Autodesk Inventor part; units mm, degrees
ref_plane "YZ Plane" through (0, 0, 0) normal (1, 0, 0) x (0, 1, 0)
ref_plane "XZ Plane" through (0, 0, 0) normal (0, 1, 0) x (-1, 0, 0)
ref_plane "XY Plane" through (0, 0, 0) normal (0, 0, 1) x (1, 0, 0)
sketch "Sketch1" plane through (0, 0, 0) normal (0, 1, 0) x (-1, 0, 0)
  line L0 (0, 0) -> (-27, 0) construction
  line L1 (-27, -8) -> (0, -8)
  arc A0 (0, -8) -> (0, 8) centre (0, 0) ccw
  arc A1 (-27, 8) -> (-27, -8) centre (-27, 0) ccw
  line L2 (14.5, 10) -> (-41.5, 10)
  line L3 (-41.5, 10) -> (-41.5, -10)
  line L4 (-41.5, -10) -> (14.5, -10)
  line L5 (14.5, -10) -> (14.5, 10)
  line L6 (14.5, 10) -> (-41.5, -10) construction
  line L7 (-41.5, 10) -> (14.5, -10) construction
  line L8 (14.5, 10) -> (-41.5, 10)
  line L9 (-41.5, 10) -> (-41.5, 15)
  line L10 (-41.5, 15) -> (14.5, 15)
  line L11 (14.5, 15) -> (14.5, 10)
  arc A2 (0, -8) -> (-5.3358, 5.9607) centre (0, 0) ccw
  arc A3 (-21.6642, 5.9607) -> (-27, -8) centre (-27, 0) ccw
  line L12 (9, -10) -> (-36, -10)
  line L13 (-36, -10) -> (-36, 10) construction
  line L14 (-36, 10) -> (9, 10)
  line L15 (9, 10) -> (9, -10) construction
  line L16 (9, -10) -> (-36, 10) construction
  line L17 (-36, -10) -> (9, 10) construction
  line L18 (9, 10) -> (-6, 10)
  line L19 (-6, 10) -> (-6, 5.9607)
  line L20 (-36, 10) -> (-21, 10)
  line L21 (-21, 10) -> (-21, 5.9607)
  line L22 (-5.3358, 5.9607) -> (-21.6642, 5.9607) construction
  line L23 (-21, 5.9607) -> (-21.6642, 5.9607)
  line L24 (-6, 5.9607) -> (-5.3358, 5.9607)
  point P0 (-13.5, 0)
  point P1 (-27, 8)
  point P2 (0, 8)
  dimension "d0" = 27
  dimension "d1" = 16
  dimension "d2" = 56
  dimension "d3" = 20
  dimension "d4" = 5
  dimension "d5" = 45
  dimension "d6" = 15
  dimension "d7" = 15
extrude "Extrusion1" add sketch "Sketch1" along normal blind 8 contours L1 A0 A2 L24 L19 L2 L5 L4 L3 L21 L23 A3 A1
extrude "Extrusion2" add sketch "Sketch1" along normal blind 15.5 contours L2 L9 L10 L11
sketch "Sketch2" plane through (21, 0, 10) normal (0, 0, -1) x (-1, 0, 0)
  line L0 (35.5, 8) -> (15, 8)
  line L1 (-20.5, 8) -> (-20.5, 15.5)
  line L2 (35.5, 8) -> (-20.5, 8)
  line L3 (-20.5, 8) -> (-20.5, 15.5)
  line L4 (-20.5, 15.5) -> (35.5, 15.5)
  line L5 (35.5, 15.5) -> (35.5, 8)
  line L6 (31, 8) -> (-16, 8)
  line L7 (-16, 8) -> (-16, 12.5)
  line L8 (-16, 12.5) -> (31, 12.5)
  line L9 (31, 12.5) -> (31, 8)
  line L10 (-20.5, 8) -> (35.5, 8)
  point P0 (21, 0)
  point P1 (7.5, 8)
  dimension "d12" = 47
  dimension "d13" = 4.5
extrude "Extrusion3" add sketch "Sketch2" along normal blind 3 contours L0 L9 L8 L7 L2 L1 L4 L5
sketch "Sketch3" plane through (41.5, 0, -10) normal (0, 0, -1) x (-1, 0, 0)
  circle A0 centre (52, 4) radius 2.15
  line L0 (56, 0) -> (56, 8)
  line L1 (0, 0) -> (56, 0)
  circle A1 centre (4, 4) radius 2.15
  line L2 (0, 0) -> (0, 8)
  point P0 (41.5, 0)
  dimension "d16" = 4.3
  dimension "d17" = 4
  dimension "d18" = 4
  dimension "d19" = 4.3
  dimension "d20" = 4
  dimension "d21" = 4
extrude "Extrusion4" cut sketch "Sketch3" against normal blind 32
sketch "Sketch4" plane through (-14.5, 0, 15) normal (0, 0, 1) x (1, 0, 0)
  circle A0 centre (4, 12) radius 1.95
  circle A1 centre (4, 4) radius 2.15
  line L0 (0, 0) -> (0, 15.5)
  circle A2 centre (52, 12) radius 1.95
  circle A3 centre (52, 4) radius 2.15
  line L1 (56, 0) -> (56, 15.5)
  line L2 (0, 15.5) -> (56, 15.5)
  point P0 (14.5, 0)
  dimension "d24" = 3.9
  dimension "d25" = 8
  dimension "d26" = 4
  dimension "d27" = 3.9
  dimension "d28" = 8
  dimension "d29" = 4
  dimension "d30" = 3.5
  dimension "d31" = 3.5
extrude "Extrusion5" add sketch "Sketch4" along normal blind 2 contours A0 | A2
sketch "Sketch5" plane through (0, 15.5, 0) normal (0, 1, 0) x (1, 0, 0)
  line L0 (-14.5, 10) -> (-14.5, -7)
  line L1 (-14.5, 0) -> (41.5, 0)
  line L2 (41.5, 0) -> (41.5, -17)
  line L3 (41.5, -17) -> (-14.5, -17)
  line L4 (-14.5, -17) -> (-14.5, 0)
  point P0 (0, 0)
  dimension "d34" = 17
extrude "Extrusion6" cut sketch "Sketch5" against normal blind 27
properties part number "Ultrasonic_sensor_frame_Top"
The listing builds one solid part. Answer for the finished solid, in the listing's coordinates (mm). A direction names the side the tool comes from. Coordinates: 2 decimals unless noted, no trailing zeros. Write each loop counter-clockwise with the first axis right and the second up, starting at its lowest first coordinate (ties: lowest second). Pieces come first, ordered by that corner, then holes. Notation, with made-up numbers: (82.5, 16) - (107.5, 16) arc R12 cw to (107.5, 37) - close; hole circle Ø4 at (56.5, 19.5). An arc over 180 degrees is marked (long way). Return JSON: item names as keys, results as strings. Group by question number.
1. Which of the six approach directions +Z, -Z, +X, -X, +Y, -Y give full straight-line access (tool end or side, diameter ignored) to faces 1 (the cylindrical face through (-5.719, 3.944, -5.594)), 2 (the cylindrical face through (35.45, 4.65, -5.07))?
2. A cutting plane is placed at D-D, the plane y = 7.25. Determine the outline of the cut face in (x, z), plus the area to 3 significant figures.
3. A cutting plane is placed at A-A, the plane y = 4. Determine the outline of the cut face in (x, z).
4. Determine the mould class of faces 3 (the flat face through (41.5, 4, -5)), 4 (the flat face through (-14.5, 4, -5)), 5 (the flat face through (40, 3, 0)), 6 (the flat face through (14, 4, -8)) for opening direction X: released by +X, released by -X, zero draft, split by the parting line, or undercut.
5. A cutting plane is placed at B-B, the plane x = -10.5. Determine the outline of the cut face in (y, z).
6. Straight lines are drawn through the part: L1, parallel to Y at x = 37.5, z = -5; L2, parallel to X at y = 3.5, z = -2.5; L3, parallel to Z at x = 22.5, y = 4. For each, find the intervals that lie inside material, in ascending order.
7. Given pin 1 (4 mm diameter, centred on x = 37.5, y = 4, fed in from -Z); pin 2 (3 mm diameter, centred on x = 7.5, y = 1, fed in from +Z), each flat-ended and moving along its own axis, determine where each tip first touches the part or whether it passes through.
8. A cutting plane is placed at C-C, the plane z = -3.75. Determine the outline of the cut face in (x, y).
Ans:
{
 "1": {"face 1": "+Z, +Y, -Y", "face 2": "+Z, -Z"},
 "2": {"outline": "(-14.5, -10) - (41.5, -10) - (41.5, 0) - (35, 0) arc R8 cw to (27, -8) - (0, -8) arc R8 cw to (-8, 0) - (-14.5, 0) - close", "area": "243 mm²"},
 "3": {"outline": "(-14.5, -10) - (-12.65, -10) - (-12.65, 0) - (-14.5, 0) - close; (-8.35, -10) - (35.35, -10) - (35.35, 0) - (35, 0) arc R8 cw to (27, -8) - (0, -8) arc R8 cw to (-8, 0) - (-8.35, 0) - close; (39.65, -10) - (41.5, -10) - (41.5, 0) - (39.65, 0) - close"},
 "4": {"face 3": "released by +X", "face 4": "released by -X", "face 5": "zero draft", "face 6": "undercut"},
 "5": {"outline": "(0, -10) - (1.85, -10) - (1.85, 0) - (0, 0) - close; (6.15, -10) - (8, -10) - (8, 0) - (6.15, 0) - close"},
 "6": {"L1": "0 to 1.85, 6.15 to 8", "L2": "-14.5 to -12.59, -8.41 to -7.6, 34.6 to 35.41, 39.59 to 41.5", "L3": "-10 to -8"},
 "7": {"pin 1": "through", "pin 2": "z = -8"},
 "8": {"outline": "(-14.5, 0) - (-7.07, 0) - (-7.07, 8) - (-14.5, 8) - close; (34.07, 0) - (41.5, 0) - (41.5, 8) - (34.07, 8) - close; hole circle Ø4.3 at (-10.5, 4); hole circle Ø4.3 at (37.5, 4)"}
}
